Part model, mm, in its own coordinate system. Face numbers are marked on the shaded views. A direction names the side the tool comes from. Round coordinates to 2 decimals unless told otherwise and drop trailing zeros. Write each loop counter-clockwise with the first axis right and the second up, starting at its lowest first coordinate (ties: lowest second). Pieces come first, ordered by that corner, then holes.
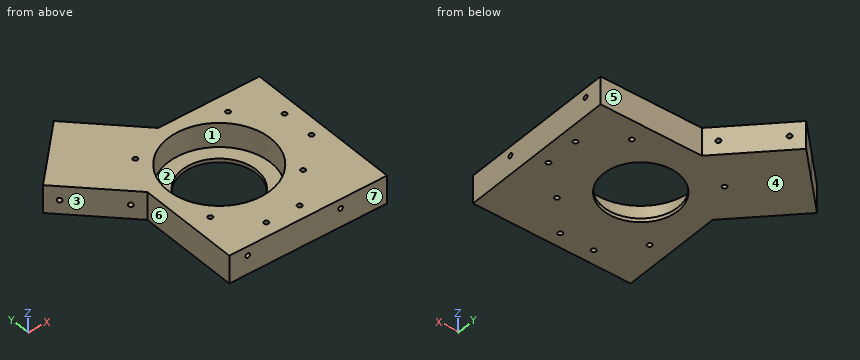
```python
from build123d import *

# Parameters (mm, degrees)
SKETCH1_R           = 27.7
SKETCH1_R_2         = 1.25
BOSS_EXTRUDE1_DEPTH = 15
CUT_EXTRUDE1_REACH  = 107.304
SKETCH2_R           = 1.25
SKETCH6_R           = 27.7
SKETCH6_R_2         = 20
BOSS_EXTRUDE4_DEPTH = 2
SKETCH7_R           = 1.25
CUT_EXTRUDE2_DEPTH  = 15
SKETCH8_R           = 1.25
CUT_EXTRUDE3_DEPTH  = 15


with BuildPart() as part:
    # Sketch1 → Boss-Extrude1 (new body)
    with BuildSketch(Plane.XY):
        Polygon((50, 35), (50, -50), (-35, -50), (-35, 4.594408409), (-66.114484041, 35.70889245), (-50.911688245, 50.911688245), (-35.70889245, 66.114484041), (-4.594408409, 35), align=None)
        Circle(SKETCH1_R, mode=Mode.SUBTRACT)
        with Locations((-25, 25)):
            Circle(SKETCH1_R_2, mode=Mode.SUBTRACT)
        with Locations((25, 25)):
            Circle(SKETCH1_R_2, mode=Mode.SUBTRACT)
        with Locations((25, -25)):
            Circle(SKETCH1_R_2, mode=Mode.SUBTRACT)
        with Locations((-25, -25)):
            Circle(SKETCH1_R_2, mode=Mode.SUBTRACT)
        with Locations((42.5, 9)):
            Circle(SKETCH1_R_2, mode=Mode.SUBTRACT)
        with Locations((42.5, -9)):
            Circle(SKETCH1_R_2, mode=Mode.SUBTRACT)
        with Locations((9, -42.5)):
            Circle(SKETCH1_R_2, mode=Mode.SUBTRACT)
        with Locations((-9, -42.5)):
            Circle(SKETCH1_R_2, mode=Mode.SUBTRACT)
    extrude(amount=BOSS_EXTRUDE1_DEPTH)

    # Sketch2 → Cut-Extrude1 (cut, up to next)
    with BuildSketch(Plane(origin=(-15.202795796, -15.202795796, 0), x_dir=(0, 0, 1), z_dir=(-0.7071067811865472, -0.7071067811865478, 0)), mode=Mode.PRIVATE) as cut_extrude1_sk1:
        with Locations(Location((7.5, 65, 0), (0, 0, 270))):
            Circle(SKETCH2_R)
    cut_extrude1_tool1 = extrude(cut_extrude1_sk1.sketch, amount=-CUT_EXTRUDE1_REACH, mode=Mode.PRIVATE) & part.part
    # Sketch2 → Cut-Extrude1 (cut, up to next)
    with BuildSketch(Plane(origin=(-15.202795796, -15.202795796, 0), x_dir=(0, 0, 1), z_dir=(-0.7071067811865472, -0.7071067811865478, 0)), mode=Mode.PRIVATE) as cut_extrude1_sk2:
        with Locations(Location((7.5, 35, 0), (0, 0, 270))):
            Circle(SKETCH2_R)
    cut_extrude1_tool2 = extrude(cut_extrude1_sk2.sketch, amount=-CUT_EXTRUDE1_REACH, mode=Mode.PRIVATE) & part.part
    add(cut_extrude1_tool1.solids().sort_by_distance((-61.164737, 30.759145, 7.5))[0], mode=Mode.SUBTRACT)
    add(cut_extrude1_tool2.solids().sort_by_distance((-39.951533, 9.545942, 7.5))[0], mode=Mode.SUBTRACT)

    # Sketch6 → Boss-Extrude4 (add)
    with BuildSketch(Plane(origin=(0, 0, 0), x_dir=(-1, 0, 0), z_dir=(0, 0, -1))):
        Circle(SKETCH6_R)
        Circle(SKETCH6_R_2, mode=Mode.SUBTRACT)
    extrude(amount=-BOSS_EXTRUDE4_DEPTH)

    # Sketch7 → Cut-Extrude2 (cut)
    with BuildSketch(Plane.XZ.offset(50)):
        with Locations((25, 10)):
            Circle(SKETCH7_R)
        with Locations((-25, 10)):
            Circle(SKETCH7_R)
    extrude(amount=-CUT_EXTRUDE2_DEPTH, mode=Mode.SUBTRACT)

    # Sketch8 → Cut-Extrude3 (cut)
    with BuildSketch(Plane(origin=(50, 0, 0), x_dir=(0, 0, -1), z_dir=(1, 0, 0))):
        with Locations(Location((-10, -25, 0), (0, 0, 90))):
            Circle(SKETCH8_R)
        with Locations(Location((-10, 25, 0), (0, 0, 90))):
            Circle(SKETCH8_R)
    extrude(amount=-CUT_EXTRUDE3_DEPTH, mode=Mode.SUBTRACT)


solid = part.part
```
Q1. Drop flat-ended pins along their axis: pin 1 (1.2 mm diameter, centred on y = 25, z = 10, fed in from +X); pin 2 (3 mm diameter, centred on x = 25, z = 10, fed in from +Y); pin 3 (3 mm diameter, centred on y = -10, z = 4.5, fed in from -X). Give the stop position or say it passes through.
Values follow:
pin 1: stops at x = 35
pin 2: stops at y = 35
pin 3: stops at x = -35
Q2. Cut at C-C on z = 13.5. State how many separate pieces and enclosed holes the cut face has, plus the area to 3 significant figures.
Values follow:
separate pieces: 1
enclosed holes: 9
area: 6,210 mm2
Q3. Cut at A-A on y = 0. Write the cut outline in (x, z), plus the area to 3 significant figures.
Values follow:
outline: (-35, 0) - (-20, 0) - (-20, 2) - (-27.7, 2) - (-27.7, 15) - (-35, 15) - close; (20, 0) - (50, 0) - (50, 15) - (27.7, 15) - (27.7, 2) - (20, 2) - close
area: 475 mm2
Q4. Which spindle directions (+Z, -Z, +X, -X, +Y, -Y) get a long thin tool onto all of the face, cutting with end or side? Do the marked faces 5, 6 and 7. Say none if no direction does.
Values follow:
face 5: +Z, -Z, +X, +Y
face 6: +Z, -Z, -X, -Y
face 7: +Z, -Z, +X, -X, -Y
Q5. Mould opens along X. For the marked faces 1, 2, 3 and 4 say: +X half, -X half, draft (parallel to the pull), parting line (faces both ways), or undercut.
Values follow:
face 1: undercut
face 2: undercut
face 3: -X half
face 4: draft
Q6. Cut at B-B on x = 0. Write the cut outline in (y, z), plus the area to 3 significant figures.
Values follow:
outline: (-50, 0) - (-20, 0) - (-20, 2) - (-27.7, 2) - (-27.7, 15) - (-50, 15) - close; (20, 0) - (35, 0) - (35, 15) - (27.7, 15) - (27.7, 2) - (20, 2) - close
area: 475 mm2
Q7. Wall check: L1, parallel to Y at x = 42.5, z = 5; L2, parallel to Y at x = -24, z = 8.5; L3, parallel to Y at x = 10, z = 13.5. Give the ranges that are in metal, low to high.
Values follow:
L1: y = -50 to -10.25, -7.75 to 7.75, 10.25 to 35
L2: y = -50 to -25.75, -24.25 to -13.83, 13.83 to 24.25, 26.56 to 54.41
L3: y = -50 to -43.25, -41.75 to -25.83, 25.83 to 35
